Study the drawing (mm; zero at the part's minimum x, y, z) and answer. A direction names the side the tool comes from. Coordinates: 2 decimals unless noted, no trailing zeros. Loops run counter-clockwise (first coordinate to the right, second up) from the corner with the lowest first, then second, coordinate; pieces in that order, holes last. Notation, with made-up numbers: M 18.25,52.25 L 57.25,52.25 A15 ccw 57.25,79.25 Z; hole C -25.5,0 d1. An arc over 180 degrees is marked long. Use one line per item in the form item = value. Start each with the question number.
1. Find the intervals of material crossed by probe 1 along Y at (x, z) = (97, 28); probe 2 along Z at (x, y) = (77, 54), in increasing order. Write a range as [from, to].
2. A tool of negligible diameter and unlimited length cuts with its end or side. For the marked faces 1 and 2, from which of +Z, -Z, +X, -X, +Y, -Y can it reach the whole face along a straight path? Write none if from no direction.
3. The part is cut by section B-B (x = 14.5). Give the vertices of the cut face in (y, z).
4. The part is cut by section A-A (z = 40). Give the vertices of the cut face in (x, y).
5. For a pull along X with two mould halves and no side action, classify the marked faces 3, 4 and 5 as released by +X, released by -X, zero draft, split by the parting line, or undercut.
6. Flat-ended cylindrical pins translate along their axes: pin 1 (8 mm diameter, centred on y = 42, z = 28.5, fed in from -X); pin 2 (1.2 mm diameter, centred on x = 101.5, z = 46.5, fed in from -Y); pin 3 (12 mm diameter, centred on x = 58.5, y = 92.5, fed in from +Z); pin 4 (3 mm diameter, centred on x = 84.5, z = 59.5, fed in from +Y). Find the tip coordinate at first contact, or state that the pin passes through.
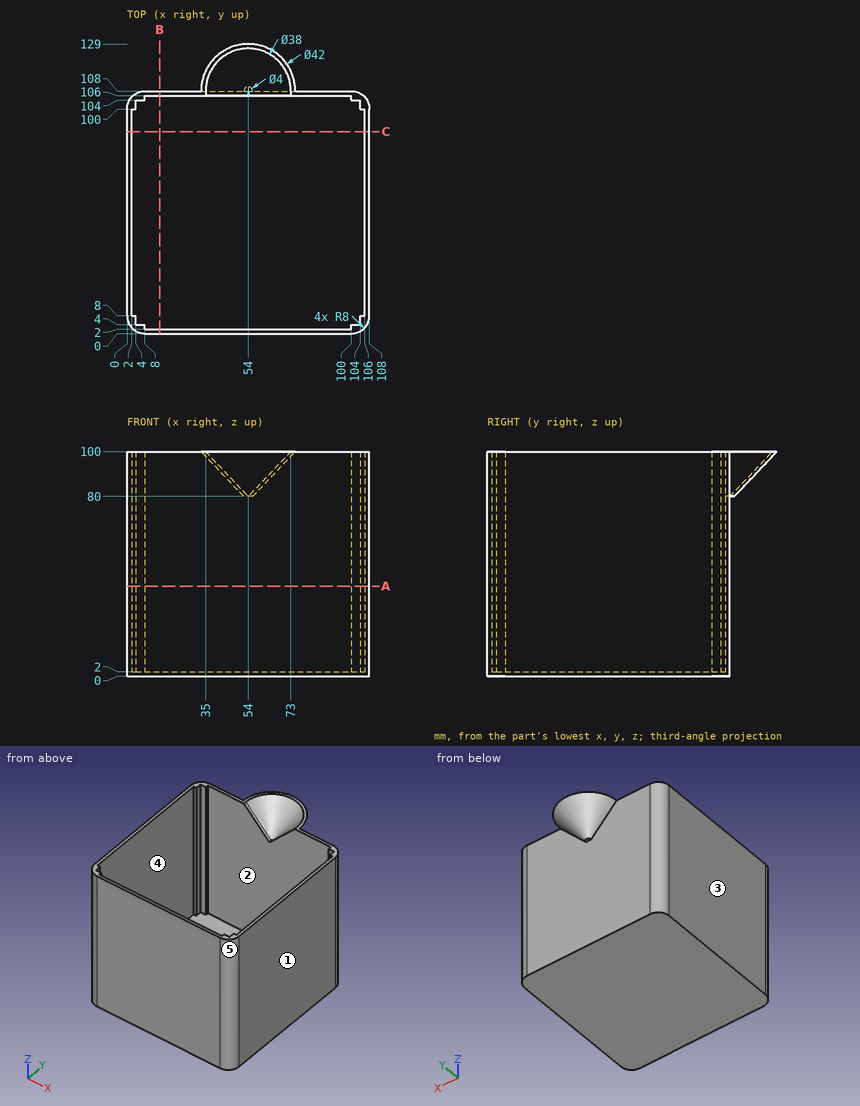
Computed values:
q1.probe_1 = [0, 2], [106, 108]
q1.probe_2 = [0, 2]
q2.face_1 = +Z, -Z, +X, +Y, -Y
q2.face_2 = +Z
q3.outline = M 0,0 L 108,0 L 108,100 L 106,100 L 106,2 L 2,2 L 2,100 L 0,100 Z
q4.outline = M 0,8 A8 ccw 8,0 L 100,0 A8 ccw 108,8 L 108,100 A8 ccw 100,108 L 8,108 A8 ccw 0,100 Z; hole M 2,8 L 4,8 L 4,4 L 8,4 L 8,2 L 100,2 L 100,4 L 104,4 L 104,8 L 106,8 L 106,100 L 104,100 L 104,104 L 100,104 L 100,106 L 8,106 L 8,104 L 4,104 L 4,100 L 2,100 Z
q5.face_3 = released by -X
q5.face_4 = undercut
q5.face_5 = released by +X
q6.pin_1 = 0
q6.pin_2 = 0.05
q6.pin_3 = 2
q6.pin_4 = 108
